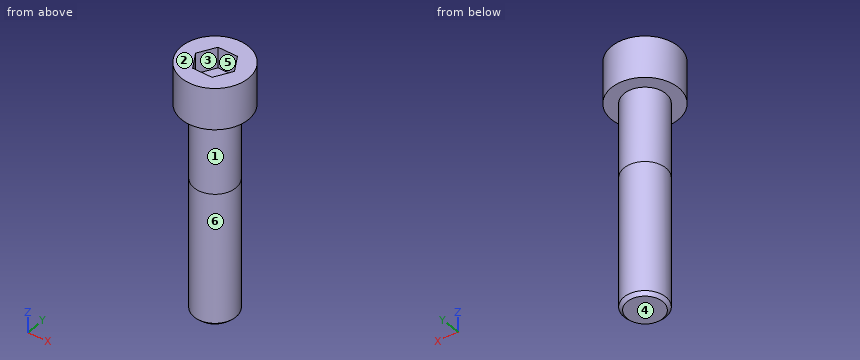
Solid Edge part; units mm, degrees
sketch "Sketch1" plane through (0, 0, 0) normal (0, 0, 1) x (1, 0, 0)
  circle A0 centre (0, 0) radius 8
extrude "Protrusion1" add sketch "Sketch1" along normal blind 10
sketch "Sketch2" plane through (0, 0, 0) normal (0, 0, -1) x (1, 0, 0)
  circle A0 centre (0, 0) radius 5
extrude "Protrusion2" add sketch "Sketch2" along normal blind 50
sketch "Sketch3" plane through (0, 0, -50) normal (0, 0, -1) x (1, 0, 0)
  circle A0 centre (0, 0) radius 4.9997
extrude "Cutout1" cut sketch "Sketch3" against normal blind 32 flip side to cut
chamfer "Chamfer_1" distance 0.75 angle 45 1 edges at (-4.9997, 0, -50)
sketch "Sketch4" plane through (0, 0, 10) normal (0, 0, 1) x (1, 0, 0)
  line L0 (-2.3094, 4) -> (2.3094, 4)
  line L1 (4.6188, 0) -> (2.3094, 4)
  line L2 (2.3094, -4) -> (4.6188, 0)
  line L3 (-2.3094, -4) -> (2.3094, -4)
  line L4 (-4.6188, 0) -> (-2.3094, -4)
  line L5 (-2.3094, 4) -> (-4.6188, 0)
extrude "Cutout2" cut sketch "Sketch4" against normal blind 5
properties part number "119167" material "Stainless Steel, 304"
Input: part model. Units: mm. Frame: model coordinates. Face numbers are marked on the shaded views. A direction names the side the tool comes from. Give positions to 0.01 mm unless a question says otherwise; leave off trailing zeros. Order: outer loops, then holes, each group sorted by start corner. A loop starts at its lowest first (then second) coordinate and runs counter-clockwise, first axis right, second up. Notation, with made-up numbers: M 35,8.5 L 39,8.5 A22 cw 39,46.5 Z; hole C -33,5 d5. An arc over 180 degrees is marked long. Return JSON: item names as keys, results as strings.
1) Mould query, pull axis Y, two halves, no side actions, for the marked faces 1, 2 and 3. Classes: released by +Y, released by -Y, zero draft, split by the parting line, or undercut.
Taken from the geometry:
{"face 1": "split by the parting line", "face 2": "zero draft", "face 3": "undercut"}
2) Contact query for flat-ended pins moving along their axis: pin 1 (2.5 mm diameter, centred on x = -1.5, y = -1.5, fed in from +Z); pin 2 (5 mm diameter, centred on y = -0.5, z = -40.5, fed in from -X); pin 3 (2 mm diameter, centred on y = 4.5, z = -21.5, fed in from +X); pin 4 (8 mm diameter, centred on x = -0.5, z = 0, fed in from +Y). Output: stop coordinate, or through.
Taken from the geometry:
{"pin 1": "stops at z = 5", "pin 2": "stops at x = -5", "pin 3": "stops at x = 3.57", "pin 4": "stops at y = 8"}
3) Section query C-C on y = 5.75. Output: boundary loops of the cut face in (x, z).
Taken from the geometry:
{"outline": "M -5.56,0 L 5.56,0 L 5.56,10 L -5.56,10 Z"}
4) Access query for the marked faces 4, 5 and 6. Directions: +Z, -Z, +X, -X, +Y, -Y. A direction counts if a zero-diameter tool reaches every point of the face in a straight line with its end or side. Return the directions, or none.
Taken from the geometry:
{"face 4": "-Z, +X, -X, +Y, -Y", "face 5": "+Z", "face 6": "-Z"}
5) Section query B-B on z = -26. Output: boundary loops of the cut face in (x, y).
Taken from the geometry:
{"outline": "C 0,0 d10"}
6) Line query: L1, parallel to Z at x = 2.75, y = 5; L2, parallel to Z at x = 0.25, y = -3.5; L3, parallel to X at y = 5.5, z = 2. Output: solid intervals per line, ascending. Write a range as [from, to].
Taken from the geometry:
{"L1": "z = [0, 10]", "L2": "z = [-50, 5]", "L3": "x = [-5.81, 5.81]"}
